Can you work these out from the model? Positions are in its coordinate system, mm. Give positions to 0.01 mm unless a question says otherwise; leave off trailing zeros. Loops run counter-clockwise (first coordinate to the right, second up) from the corner with the lowest first, then second, coordinate; pieces in that order, holes last. Notation, with made-up numbers: M 62.5,61.25 L 75.5,61.25 A14 ccw 75.5,82.25 Z; hole C -32,-24.75 d10. An arc over 180 degrees is marked long. Use CSV: the item, a comma, the result in double quotes.
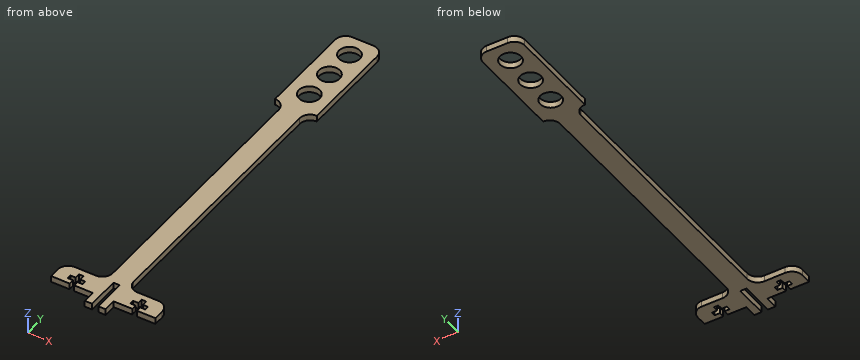
from build123d import *

# Parameters (mm, degrees)
SKETCH1_R           = 5
BOSS_EXTRUDE1_DEPTH = 3
FILLET1_START       = -1
FILLET1_DEPTH       = 5
FILLET1_2_DEPTH     = 3


with BuildPart() as part:
    # Sketch1 → Boss-Extrude1 (new body)
    with BuildSketch(Plane.XY):
        Polygon((-5, -25), (-5, -159), (-25, -159), (-25, -169), (-16.1, -169), (-16.1, -166.5), (-18.6, -166.5), (-18.6, -164.5), (-16.1, -164.5), (-16.1, -162), (-13.9, -162), (-13.9, -164.5), (-11.4, -164.5), (-11.4, -166.5), (-13.9, -166.5), (-13.9, -169), (-5, -169), (-5, -175), (-1.5, -175), (-1.5, -159), (1.5, -159), (1.5, -175), (5, -175), (5, -169), (13.9, -169), (13.9, -166.5), (11.4, -166.5), (11.4, -164.5), (13.9, -164.5), (13.9, -162), (16.1, -162), (16.1, -164.5), (18.6, -164.5), (18.6, -166.5), (16.1, -166.5), (16.1, -169), (25, -169), (25, -159), (5, -159), (5, -25), (10, -25), (10, 25), (-10, 25), (-10, -25), align=None)
        with Locations((0, 15)):
            Circle(SKETCH1_R, mode=Mode.SUBTRACT)
        Circle(SKETCH1_R, mode=Mode.SUBTRACT)
        with Locations((0, -15)):
            Circle(SKETCH1_R, mode=Mode.SUBTRACT)
    extrude(amount=BOSS_EXTRUDE1_DEPTH)

    # Fillet1: read off the stored shape, not the designer's step
    # Fillet1 outline → Fillet1 (cut)
    with BuildSketch(Plane.XY.offset(FILLET1_START)):
        with BuildLine():
            Line((25, -159), (20, -159))
            ThreePointArc((20, -159), (23.535533906, -160.464466094), (25, -164))
            Line((25, -164), (25, -159))
        make_face()
        with BuildLine():
            ThreePointArc((-25, -164), (-23.535533906, -160.464466094), (-20, -159))
            Line((-20, -159), (-25, -159))
            Line((-25, -159), (-25, -164))
        make_face()
        with BuildLine():
            ThreePointArc((-10, 20), (-8.535533906, 23.535533906), (-5, 25))
            Line((-5, 25), (-10, 25))
            Line((-10, 25), (-10, 20))
        make_face()
        with BuildLine():
            ThreePointArc((5, 25), (8.535533906, 23.535533906), (10, 20))
            Line((10, 20), (10, 25))
            Line((10, 25), (5, 25))
        make_face()
    extrude(amount=FILLET1_DEPTH, mode=Mode.SUBTRACT)

    # Fillet1 2 outline → Fillet1 2 (add)
    with BuildSketch(Plane.XY):
        with BuildLine():
            Line((-5, -159), (-5, -154))
            ThreePointArc((-5, -154), (-6.464466094, -157.535533906), (-10, -159))
            Line((-10, -159), (-5, -159))
        make_face()
        with BuildLine():
            Line((-5, -25), (-10, -25))
            ThreePointArc((-10, -25), (-6.464466094, -26.464466094), (-5, -30))
            Line((-5, -30), (-5, -25))
        make_face()
        with BuildLine():
            Line((5, -25), (5, -30))
            ThreePointArc((5, -30), (6.464466094, -26.464466094), (10, -25))
            Line((10, -25), (5, -25))
        make_face()
        with BuildLine():
            Line((5, -159), (10, -159))
            ThreePointArc((10, -159), (6.464466094, -157.535533906), (5, -154))
            Line((5, -154), (5, -159))
        make_face()
    extrude(amount=FILLET1_2_DEPTH)


solid = part.part
Q1. I'm going to push flat-ended pins straight in: P1, Ø4, axis at x = -1, y = -152, coming from the -Z side; P2, Ø0.7, axis at x = 15.5, z = 1, coming from the -Y side; P3, Ø0.9, axis at x = 19, z = 1, coming from the -Y side. Where does each tip first touch, or does it pass through?
Model answer:
P1,"z = 0"
P2,"y = -162"
P3,"y = -169"
Q2. I want a section at C-C, the plane y = -42.5. Please give me the cut outline in (x, z), then the cut area to 3 significant figures.
Model answer:
outline,"M -5,0 L 5,0 L 5,3 L -5,3 Z"
area,"30.0 mm2"
Q3. I want a section at A-A, the plane y = 15. Please give me the cut outline in (x, z), then the cut area to 3 significant figures.
Model answer:
outline,"M -10,0 L -5,0 L -5,3 L -10,3 Z; M 5,0 L 10,0 L 10,3 L 5,3 Z"
area,"30.0 mm2"
Q4. I want a section at B-B, the plane z = 1.6. State how many separate pieces and enclosed holes the cut face has, then the cut area to 3 significant figures.
Model answer:
separate pieces,"1"
enclosed holes,"3"
area,"2,570 mm2"
Q5. Please list where these lines run through material, in increasing order: L1, parallel to Y at x = 0, z = 1.45; L2, parallel to X at y = -38, z = 0.2; L3, parallel to Y at x = 2, z = 1.8. Write a range as from..to.
Model answer:
L1,"-159..-20, -10..-5, 5..10, 20..25"
L2,"-5..5"
L3,"-175..-19.58, -10.42..-4.58, 4.58..10.42, 19.58..25"
